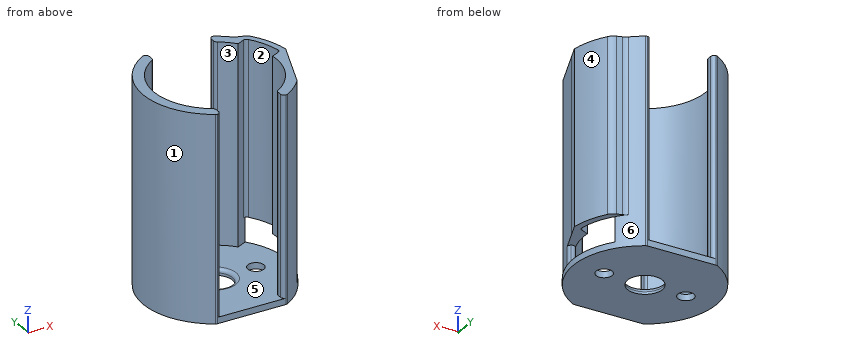
```python
from build123d import *

# Parameters (mm, degrees)
SKETCH1_R           = 14.605
SKETCH1_R_2         = 12.446
BOSS_EXTRUDE1_DEPTH = 40.64
BOSS_EXTRUDE2_START = 1.27
SKETCH2_R           = 14.605
SKETCH2_R_2         = 3.556
SKETCH2_R_3         = 1.651
BOSS_EXTRUDE2_DEPTH = 1.27
SKETCH3_W           = 34.056453184
SKETCH3_H           = 6.418177278
SKETCH3_W_2         = 34.979066167
SKETCH3_H_2         = 5.575791511
CUT_EXTRUDE1_DEPTH  = 47.723229233
SKETCH4_W           = 12.7
SKETCH4_H           = 40.64
CUT_EXTRUDE2_DEPTH  = 51.100654936
CUT_EXTRUDE3_DEPTH  = 40.64
BOSS_EXTRUDE3_DEPTH = 41.91
SKETCH7_R           = 15.875
SKETCH7_R_2         = 14.605
CUT_EXTRUDE4_DEPTH  = 6.35
CUT_EXTRUDE5_DEPTH  = 5.08
CUT_EXTRUDE6_REACH  = 48.533
BOSS_EXTRUDE5_DEPTH = 35.56
FILLET1_R           = 0.762
FILLET2_R           = 2.54


with BuildPart() as part:
    # Sketch1 → Boss-Extrude1 (new body)
    with BuildSketch(Plane.XY):
        Circle(SKETCH1_R)
        Circle(SKETCH1_R_2, mode=Mode.SUBTRACT)
    extrude(amount=BOSS_EXTRUDE1_DEPTH)

    # Sketch2 → Boss-Extrude2 (add)
    with BuildSketch(Plane(origin=(0, 0, 0), x_dir=(-1, 0, 0), z_dir=(0, 0, -1)).offset(BOSS_EXTRUDE2_START)):
        Circle(SKETCH2_R)
        Circle(SKETCH2_R_2, mode=Mode.SUBTRACT)
        with Locations((-8.382, 0)):
            Circle(SKETCH2_R_3, mode=Mode.SUBTRACT)
        with Locations((8.382, 0)):
            Circle(SKETCH2_R_3, mode=Mode.SUBTRACT)
    extrude(amount=-BOSS_EXTRUDE2_DEPTH)

    # Sketch3 → Cut-Extrude1 (cut, through all)
    with BuildSketch(Plane(origin=(0, 0, -1.27), x_dir=(-1, 0, 0), z_dir=(0, 0, -1))):
        with Locations((0.581647316, 15.909088639)):
            Rectangle(SKETCH3_W, SKETCH3_H)
        with Locations((1.042953807, -15.487895756)):
            Rectangle(SKETCH3_W_2, SKETCH3_H_2)
    extrude(amount=-CUT_EXTRUDE1_DEPTH, mode=Mode.SUBTRACT)

    # Sketch4 → Cut-Extrude2 (cut, through all)
    with BuildSketch(Plane(origin=(0, 12.7, 0), x_dir=(1, 0, 0), z_dir=(0, 1, 0))):
        with Locations((0, -20.32)):
            Rectangle(SKETCH4_W, SKETCH4_H)
    extrude(amount=-CUT_EXTRUDE2_DEPTH, mode=Mode.SUBTRACT)

    # Sketch5 → Cut-Extrude3 (cut)
    with BuildSketch(Plane.XY.offset(40.64)):
        Polygon((8.706975565, 7.656948551), (15.156085268, 10.664217794), (18.376436422, 3.758152456), (11.927326719, 0.750883214), align=None)
    extrude(amount=-CUT_EXTRUDE3_DEPTH, mode=Mode.SUBTRACT)

    # Sketch6 → Boss-Extrude3 (add)
    with BuildSketch(Plane(origin=(0, 0, -1.27), x_dir=(-1, 0, 0), z_dir=(0, 0, -1))):
        with BuildLine():
            Line((-12.527218586, 9.751124012), (-10.16966665, 10.48255242))
            ThreePointArc((-10.16966665, 10.48255242), (-10.873649709, 9.75037266), (-11.525041099, 8.971034091))
            ThreePointArc((-11.525041099, 8.971034091), (-13.467409843, 5.651096984), (-14.475687068, 1.93920316))
            ThreePointArc((-14.475687068, 1.93920316), (-14.575462242, 0.928399389), (-14.604741501, -0.086894693))
            Line((-14.604741501, -0.086894693), (-15.734442466, 2.107829522))
            ThreePointArc((-15.734442466, 2.107829522), (-14.638488959, 6.142496722), (-12.527218586, 9.751124012))
        make_face()
    extrude(amount=-BOSS_EXTRUDE3_DEPTH)

    # Sketch7 → Cut-Extrude4 (cut)
    with BuildSketch(Plane(origin=(0, 0, -1.27), x_dir=(-1, 0, 0), z_dir=(0, 0, -1))):
        Circle(SKETCH7_R)
        Circle(SKETCH7_R_2, mode=Mode.SUBTRACT)
    extrude(amount=-CUT_EXTRUDE4_DEPTH, mode=Mode.SUBTRACT)

    # Sketch8 → Cut-Extrude5 (cut)
    with BuildSketch(Plane.XY):
        with BuildLine():
            Line((14.475687068, 1.93920316), (12.407758156, 0.974912072))
            ThreePointArc((12.407758156, 0.974912072), (12.445878018, -0.05510311), (12.398639212, -1.084740374))
            Line((12.398639212, -1.084740374), (14.549423566, -1.272909623))
            ThreePointArc((14.549423566, -1.272909623), (14.601153344, 0.335180604), (14.475687068, 1.93920316))
        make_face()
        with BuildLine():
            Line((14.549423566, -1.272909623), (12.398639212, -1.084740374))
            ThreePointArc((12.398639212, -1.084740374), (12.226851946, -2.325297292), (11.931259886, -3.542309069))
            Line((11.931259886, -3.542309069), (13.780666558, -4.837277563))
            ThreePointArc((13.780666558, -4.837277563), (14.276718156, -3.079179062), (14.549423566, -1.272909623))
        make_face()
    extrude(amount=CUT_EXTRUDE5_DEPTH, mode=Mode.SUBTRACT)

    # Cut-Extrude6: up to this face of the body (flat: up to its plane)
    cut_extrude6_end = Plane(part.part.faces().sort_by_distance((9.524357094, -7.422304107, 0))[0])
    # Sketch11 → Cut-Extrude6 (cut, up to the picked face)
    with BuildSketch(Plane.XY.offset(40.64), mode=Mode.PRIVATE) as cut_extrude6_sk1:
        Polygon((15.734442466, 2.107829522), (11.428920073, -9.093173867), (14.392518886, -10.232343334), (18.698041279, 0.968660056), align=None)
    cut_extrude6_tool1 = split(extrude(cut_extrude6_sk1.sketch, amount=-CUT_EXTRUDE6_REACH, mode=Mode.PRIVATE), bisect_by=cut_extrude6_end, keep=Keep.BOTH, mode=Mode.PRIVATE)
    add(cut_extrude6_tool1.solids().sort_by(Axis((15.063481, -4.062257, 40.64), (0, 0, -1)))[0], mode=Mode.SUBTRACT)

    # Sketch12 → Boss-Extrude5 (add)
    with BuildSketch(Plane.XY.offset(40.64)):
        Polygon((14.577046288, -0.903186872), (15.734442466, 2.107829522), (15.155744377, 2.330273663), (13.998348199, -0.680742731), align=None)
    extrude(amount=-BOSS_EXTRUDE5_DEPTH)

    # Fillet1
    # the kernel refuses this fillet: 0.762 mm, written as the material it adds along each edge
    with BuildSketch(Plane(origin=(14.475687068, 1.93920316, 40.64), x_dir=(-0.1526781379658876, 0.9882759666142191, 0), z_dir=(0, 0, -1))) as fillet1_piece_1:
        with BuildLine():
            CenterArc((0.57198511, -0.76184596), FILLET1_R, 88.847914045, 74.934246566)
            Line((-0.159692452, -0.549026914), (0, 0))
            ThreePointArc((0, 0), (0.29365307, 0.002952442), (0.587306139, 0))
        make_face()
    extrude(amount=35.56)
    with BuildSketch(Plane(origin=(11.525041099, 8.971034091, 40.64), x_dir=(0.5968718617370223, -0.8023365756754336, 0), z_dir=(0, 0, -1))) as fillet1_piece_2:
        with BuildLine():
            CenterArc((0.62099819, 0.761818426), FILLET1_R, 191.646188227, 79.60463439)
            Line((-0.12531439, 0.60799537), (0, 0))
            ThreePointArc((0, 0), (0.318816035, -0.00348017), (0.63763207, 0))
        make_face()
    extrude(amount=35.56)
    # the kernel refuses this fillet: 0.762 mm, written as the material it takes off along each edge
    with BuildSketch(Plane(origin=(0, 0, 0), x_dir=(-1, 0, 0), z_dir=(0, -1, 0))) as fillet1_2_piece_1:
        with BuildLine():
            CenterArc((3.556 + FILLET1_R, FILLET1_R), FILLET1_R, 180, 90)
            Line((3.556, FILLET1_R), (3.556, 0))
            Line((3.556, 0), (3.556 + FILLET1_R, 0))
        make_face()
    revolve(axis=Axis((0, 0, 0), (0, 0, -1)), mode=Mode.SUBTRACT)
    with BuildSketch(Plane(origin=(11.931259886, -3.542309069, 0), x_dir=(-0.32230782021248533, -0.9466349185561855, 0), z_dir=(0, 0, 1))) as fillet1_2_piece_2:
        with BuildLine():
            CenterArc((1.014668485, 0.761403744), FILLET1_R, 163.802549626, 103.930693134)
            Line((0.282915237, 0.973962404), (0, 0))
            ThreePointArc((0, 0), (0.492264909, 0.009738855), (0.984529818, 0))
        make_face()
    extrude(amount=5.08, mode=Mode.SUBTRACT)
    with BuildSketch(Plane(origin=(13.216640292, -4.442342119, 0), x_dir=(-0.35879353276176223, -0.9334169490899199, 0), z_dir=(0, 0, 1))) as fillet1_2_piece_3:
        with BuildLine():
            CenterArc((FILLET1_R * 0.781652785228, -FILLET1_R), FILLET1_R, 90, 76.026121217)
            Line((-FILLET1_R * 0.1887531327, -FILLET1_R * 0.758520488551), (0, 0))
            Line((0, 0), (FILLET1_R * 0.781652785228, 0))
        make_face()
    extrude(amount=5.08, mode=Mode.SUBTRACT)
    with BuildSketch(Plane(origin=(-7.212213599, 12.7, -1.794261411), x_dir=(1, 0, 0), z_dir=(0, 0, 1)), Plane(origin=(-7.212213599, -12.7, 41.164261411), x_dir=(1, 0, 0), z_dir=(0, 0, -1))) as fillet1_2_piece_4:
        with BuildLine():
            CenterArc((0.204160731, -0.762), FILLET1_R, 90, 30.414529102)
            ThreePointArc((-0.181603647, -0.104862385), (-0.090990033, -0.052105246), (0, 0))
            Line((0, 0), (0.204160731, 0))
        make_face()
    extrude(amount=42.958522823, mode=Mode.SUBTRACT)
    with BuildSketch(Plane(origin=(7.212213599, 12.7, -1.794261411), x_dir=(0.8659975867148599, -0.500048177482969, -1.8558242316030044e-14), z_dir=(0, 0, 1)), Plane(origin=(7.212213599, -12.7, 41.164261411), x_dir=(0.8659975867148587, 0.5000481774829708, -1.8313973834794986e-14), z_dir=(0, 0, -1))) as fillet1_2_piece_5:
        with BuildLine():
            CenterArc((0.204234011, -0.761980363), FILLET1_R, 89.588658346, 30.414529102)
            Line((-0.176802701, -0.102090202), (0, 0))
            ThreePointArc((0, 0), (0.104852282, 0.000376383), (0.209704565, 0))
        make_face()
    extrude(amount=42.958522823, mode=Mode.SUBTRACT)
    with BuildSketch(Plane(origin=(-6.35, 10.704224213, 41.703745389), x_dir=(0, 1, 0), z_dir=(0, 0, -1))) as fillet1_2_piece_6:
        with BuildLine():
            CenterArc((0.425498156, -0.762), FILLET1_R, 90, 57.421029607)
            ThreePointArc((-0.216601212, -0.351692308), (-0.106841566, -0.176744751), (0, 0))
            Line((0, 0), (0.425498156, 0))
        make_face()
    extrude(amount=41.703745389, mode=Mode.SUBTRACT)
    with BuildSketch(Plane(origin=(-6.35, -10.704224213, 41.703745389), x_dir=(0, -1, 0), z_dir=(0, 0, -1)), Plane(origin=(6.35, 10.704224213, 41.703745389), x_dir=(0, 1, 0), z_dir=(0, 0, -1))) as fillet1_2_piece_7:
        with BuildLine():
            CenterArc((0.425498156, 0.762), FILLET1_R, 212.578970393, 57.421029607)
            ThreePointArc((-0.216601212, 0.351692308), (-0.106841566, 0.176744751), (0, 0))
            Line((0, 0), (0.425498156, 0))
        make_face()
    extrude(amount=41.703745389, mode=Mode.SUBTRACT)
    with BuildSketch(Plane(origin=(6.35, -10.704224213, 41.703745389), x_dir=(0.8514689576122441, 0.5244050097231324, 0), z_dir=(0, 0, -1))) as fillet1_2_piece_8:
        with BuildLine():
            CenterArc((0.425685981, 0.761895088), FILLET1_R, 211.628197432, 57.421029608)
            Line((-0.223133364, 0.362298471), (0, 0))
            ThreePointArc((0, 0), (0.206520922, 0.001713556), (0.413041843, 0))
        make_face()
    extrude(amount=41.703745389, mode=Mode.SUBTRACT)
    with BuildSketch(Plane(origin=(6.35, -12.7, 42.545), x_dir=(1, 0, 0), z_dir=(0, 0, -1)), Plane(origin=(-6.35, -12.7, 0), x_dir=(-1, 0, 0), z_dir=(0, 0, 1))) as fillet1_2_piece_9:
        with BuildLine():
            CenterArc((FILLET1_R, -FILLET1_R), FILLET1_R, 90, 90)
            Line((0, -FILLET1_R), (0, 0))
            Line((0, 0), (FILLET1_R, 0))
        make_face()
    extrude(amount=42.545, mode=Mode.SUBTRACT)
    with BuildSketch(Plane(origin=(-6.35, 12.7, 0), x_dir=(-1, 0, 0), z_dir=(0, 0, 1)), Plane(origin=(6.35, 12.7, 42.545), x_dir=(1, 0, 0), z_dir=(0, 0, -1))) as fillet1_2_piece_10:
        with BuildLine():
            CenterArc((FILLET1_R, FILLET1_R), FILLET1_R, 180, 90)
            Line((0, FILLET1_R), (0, 0))
            Line((0, 0), (FILLET1_R, 0))
        make_face()
    extrude(amount=42.545, mode=Mode.SUBTRACT)

    # Fillet2
    fillet2_edges = [part.edges().sort_by_distance(p)[0] for p in [
        (12.527218586, 9.751124012, 22.86),
        (10.16966665, 10.48255242, 22.86),
    ]]
    fillet(fillet2_edges, radius=FILLET2_R)


solid = part.part
```
Here's how the part is built. I have some questions about the finished solid (model axes, mm). Face numbers are marked on the shaded views. A direction names the side the tool comes from. Round coordinates to 2 decimals unless told otherwise and drop trailing zeros. Order: outer loops, then holes, each group sorted by start corner. A loop starts at its lowest first (then second) coordinate and runs counter-clockwise, first axis right, second up. Notation, with made-up numbers: (-39, -12.5) -> (11, -12.5) arc R23 cw to (11, 22.5) -> close; hole circle Ø1 at (68, -28.5). An arc over 180 degrees is marked (long way). Use a Markdown table: item, result. Add a question column.
(1) For the marked faces 1 and 2, which set-ups out of +Z, -Z, +X, -X, +Y, -Y let a thin tool reach every point of the face, with its end or its side?
(2) Suppose I cut it at D-D, the plane y = 7. Please give me the cut outline in (x, z).
(3) Suppose I cut it at A-A, the plane x = 0. Please give me the cut outline in (y, z).
(4) If we mould it in two halves opening along Y, with no side actions, what happens to the marked faces 3, 4, 5 and 6? For each: released by +Y, released by -Y, zero draft, split by the parting line, or undercut.
(5) I need wall thicknesses on line 1 along Y through (x, z) = (0, -0.85); line 2 along Z through (x, y) = (-8, -4.5); line 3 along Y through (x, z) = (10.5, 15). Which ranges of each line are inside material? Lowest first, please.
(6) For pin 1 Ø12 at (y, z) = (-3, 36.5) entering from +X; pin 2 Ø5 at (x, y) = (0, 3.5) entering from +Z; pin 3 Ø1.5 at (y, z) = (1.5, 4.5) entering from -X, each with a flat end and sliding along its axis, tell me the tip position at first contact or that it passes through.
(7) Suppose I cut it at B-B, the plane y = 0. Please give me the cut outline in (x, z) (3 decimals), and give its area (3 significant figures).
Verdict:
| question | item | result |
|---|---|---|
| 1 | face 1 | +Z, -Z, -X |
| 1 | face 2 | +Z |
| 2 | outline | (-12.82, -1.27) -> (12.82, -1.27) -> (12.82, 0) -> (-10.29, 0) -> (-10.29, 40.64) -> (-12.82, 40.64) -> close; (12.82, 5.08) -> (14.25, 5.08) -> (14.25, 40.64) -> (12.82, 40.64) -> close |
| 3 | outline | (-12.7, -1.27) -> (-3.56, -1.27) -> (-3.56, -0.76) arc R0.76 ccw to (-4.32, 0) -> (-12.7, 0) -> close; (3.56, -1.27) -> (12.7, -1.27) -> (12.7, 0) -> (4.32, 0) arc R0.76 ccw to (3.56, -0.76) -> close |
| 4 | face 3 | undercut |
| 4 | face 4 | released by +Y |
| 4 | face 5 | undercut |
| 4 | face 6 | split by the parting line |
| 5 | line 1 | -12.7 to -3.56, 3.56 to 12.7 |
| 5 | line 2 | -1.27 to 0 |
| 5 | line 3 | -10.15 to -6.68, 8.49 to 10.39 |
| 6 | pin 1 | x = 15.73 |
| 6 | pin 2 | z = 0 |
| 6 | pin 3 | x = -14.59 |
| 7 | outline | (-14.605, -1.27) -> (-10.033, -1.27) -> (-10.033, 0) -> (-12.446, 0) -> (-12.446, 40.64) -> (-14.605, 40.64) -> close; (-6.731, -1.27) -> (-3.556, -1.27) -> (-3.556, -0.762) arc R0.762 ccw to (-4.318, 0) -> (-6.731, 0) -> close; (3.556, -1.27) -> (6.731, -1.27) -> (6.731, 0) -> (4.318, 0) arc R0.762 ccw to (3.556, -0.762) -> close; (10.033, -1.27) -> (14.605, -1.27) -> (14.605, 0) -> (10.033, 0) -> close; (12.446, 5.08) -> (14.924, 5.08) -> (14.924, 40.64) -> (12.446, 40.64) -> close |
| 7 | area | 195 mm2 |
